```python
from build123d import *

# Parameters (mm, degrees)
F1_DEPTH = 76.2
F3_DEPTH = 76.2
F5_W     = 25.4
F5_H     = 45.78858
F6_DEPTH = 25.4


with BuildPart() as f1:
    # F0 (on Right) → F1 (new body)
    with BuildSketch(Plane.YZ):
        Polygon((13.522523, 16.816804), (-11.877477, 16.816804), (-24.577477, -8.583196), (-24.577477, -33.983196), (13.522523, -33.983196), align=None)
    extrude(amount=-F1_DEPTH)

    # F2 (on face) → F3 (join)
    with BuildSketch(Plane.YZ):
        Polygon((-24.577477, -33.983196), (-24.577477, -8.583196), (-37.277477, -8.583196), (-37.277477, -21.283196), align=None)
    extrude(amount=-F3_DEPTH)

    # F5 (on face) → F6 (cut)
    with BuildSketch(Plane(origin=(0, -3.600826, 5.401239), x_dir=(1, 0, 0), z_dir=(0, -0.5547, 0.83205))):
        with Locations((-38.1, -2.316508)):
            Rectangle(F5_W, F5_H)
    extrude(amount=F6_DEPTH, mode=Mode.SUBTRACT)


solid = f1.part
```
Geometry check sheet. Reference: the model listing, model coordinates, mm. A direction names the side the tool comes from. Coordinates: 2 decimals unless noted, no trailing zeros. Order: outer loops, then holes, each group sorted by start corner. A loop starts at its lowest first (then second) coordinate and runs counter-clockwise, first axis right, second up. Notation, with made-up numbers: M 88.25,33.25 L 94.25,33.25 A18 ccw 94.25,60.25 Z; hole C 86,36.25 d11. An arc over 180 degrees is marked long. Answer as a JSON object with one key per item and string values.
Q1. Cross-section at B-B on y = 2.5. Record the cut outline in (x, z).
Results are:
{"outline": "M -76.2,-33.98 L 0,-33.98 L 0,16.82 L -25.4,16.82 L -25.4,9.47 L -50.8,9.47 L -50.8,16.82 L -76.2,16.82 Z"}
Q2. Tool access check on faces 1 (the flat face through (0, -7, -8)), 2 (the flat face through (-50.8, -8, 7)), 3 (the flat face through (-38, -31, -8.583)). Record the directions out of +Z, -Z, +X, -X, +Y, -Y that give a thin tool (end or side, any length) a straight path to the whole face; none if there is none.
Results are:
{"face 1": "+Z, -Z, +X, +Y, -Y", "face 2": "+Z, -Y", "face 3": "+Z, +X, -X, -Y"}
Q3. Cross-section at C-C on z = 9. Record the cut outline in (x, y).
Results are:
{"outline": "M -76.2,-15.79 L -50.8,-15.79 L -50.8,1.8 L -25.4,1.8 L -25.4,-15.79 L 0,-15.79 L 0,13.52 L -76.2,13.52 Z"}
Q4. Cross-section at D-D on x = -58. Record the cut outline in (y, z).
Results are:
{"outline": "M -37.28,-21.28 L -24.58,-33.98 L 13.52,-33.98 L 13.52,16.82 L -11.88,16.82 L -24.58,-8.58 L -37.28,-8.58 Z"}
Q5. Depth check by flat-ended pin: pin 1 Ø5 at (y, z) = (-4, 2) entering from +X; pin 2 Ø5 at (x, z) = (-58.5, -6) entering from -Y; pin 3 Ø12 at (x, y) = (-65, -20) entering from +Z; pin 4 Ø10 at (x, y) = (-43.5, -28.5) entering from +Z. Enter the tip coordinate at first touch or a pass-through.
Results are:
{"pin 1": "stops at x = 0", "pin 2": "stops at y = -24.54", "pin 3": "stops at z = 12.57", "pin 4": "stops at z = -7.86"}
Q6. Scan lines: line 1 (X direction, y = 4, z = 12); line 2 (Y direction, x = -17, z = -26); line 3 (Z direction, x = -4.5, y = -24). Record each from-to range of solid material in increasing order.
Results are:
{"line 1": "x = -76.2 to -50.8, -25.4 to 0", "line 2": "y = -32.56 to 13.52", "line 3": "z = -33.98 to -7.43"}
